Geometry: final body of the model. Coordinates: model frame, mm. Round coordinates to 2 decimals unless told otherwise and drop trailing zeros. Write each loop counter-clockwise with the first axis right and the second up, starting at its lowest first coordinate (ties: lowest second). Pieces come first, ordered by that corner, then holes. Notation, with made-up numbers: M -15,42 L 36,42 A29 ccw 36,79 Z; hole C -37,-35.5 d11. An arc over 180 degrees is marked long. Use one line per item in the form item = value. Start each with the question number.
Item 1: Section query D-D (y = 7.75). Return loops of the section in (x, z), and give its area (3 significant figures).
Item 2: Ray query, probe 1 along Z at (x, y) = (6, 3.5); probe 2 along Z at (x, y) = (4.25, 8). Return the intervals inside material, ascending.
Item 3: Section query B-B (z = 2.9). State how many separate pieces and enclosed holes the cut face has, and give its area (3 significant figures).
Item 4: Section query C-C (y = 2.5). Return loops of the section in (x, z).
from build123d import *

# Parameters (mm, degrees)
F0_W     = 12.7
F0_H     = 11.1125
F1_DEPTH = 6.35
F2_R     = 0.6047619048
F3_DEPTH = 12.701
F4_DEPTH = 3.175


# Not quite as in the source:
# - a length typed as a fraction of an inch, garbled in the dataset ("3 / 203.2 mm" for 3/8 in), is restored


with BuildPart() as f1:
    # F0 (on Top) → F1 (new body)
    with BuildSketch(Plane.XY):
        with Locations((6.35, 5.55625)):
            Rectangle(F0_W, F0_H)
    extrude(amount=F1_DEPTH)

    # F2 (on face) → F3 (cut, through all)
    with BuildSketch(Plane(origin=(0, 0, 0), x_dir=(0, -1, 0), z_dir=(-1, 0, 0))):
        with Locations((-10.3481481481, 3.175)):
            Circle(F2_R)
        with Locations((-8.9790343915, 3.175)):
            Circle(F2_R)
        with Locations((-7.6099206349, 3.175)):
            Circle(F2_R)
        with Locations((-6.2408068783, 3.175)):
            Circle(F2_R)
        with Locations((-4.8716931217, 3.175)):
            Circle(F2_R)
        with Locations((-3.5025793651, 3.175)):
            Circle(F2_R)
        with Locations((-2.1334656085, 3.175)):
            Circle(F2_R)
        with Locations((-0.7643518519, 3.175)):
            Circle(F2_R)
    extrude(amount=-F3_DEPTH, mode=Mode.SUBTRACT)

    # F4 (cut): a face of the model
    f4_faces = [f1.faces().sort_by_distance(p)[0] for p in [
        (6.35, 5.55625, 6.35),
    ]]
    extrude(f4_faces, amount=-F4_DEPTH, mode=Mode.SUBTRACT)


solid = f1.part
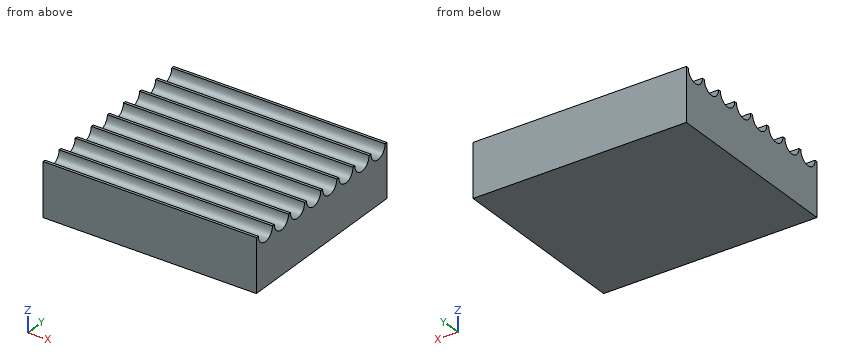
Working result:
q1.outline = M 0,0 L 12.7,0 L 12.7,2.59 L 0,2.59 Z
q1.area = 32.9 mm²
q2.probe_1 = 0 to 2.57
q2.probe_2 = 0 to 2.71
q3.separate_pieces = 9
q3.enclosed_holes = 0
q3.area = 31.7 mm²
q4.outline = M 0,0 L 12.7,0 L 12.7,2.69 L 0,2.69 Z
